Geometry: final body of the model. Coordinates: model frame, mm. A direction names the side the tool comes from. Give positions to 0.01 mm unless a question says otherwise; leave off trailing zeros. Loops run counter-clockwise (first coordinate to the right, second up) from the corner with the lowest first, then second, coordinate; pieces in that order, holes last. Notation, with made-up numbers: (-21, -31.75) -> (-3, -31.75) arc R27 ccw to (-3, -14.75) -> close; hole circle Ø1 at (67, -2.75). An arc over 180 degrees is marked (long way). One line per question, with ' | ' between items. Start each with the question number.
Item 1: Mould query, pull axis Z, two halves, no side actions, for faces 4 (the flat face through (34, -60, -4)), 5 (the flat face through (34, -77, 60)), 6 (the flat face through (50, -9, 1)), 7 (the cylindrical face through (34.255, -77.465, 50.103)). Classes: released by +Z, released by -Z, zero draft, split by the parting line, or undercut.
Item 2: Section C-C on z = 1.5. Return loops of the section in (x, y).
Item 3: Material intervals for line 1 along Z through (x, y) = (56, 8); line 2 along Y through (x, z) = (28.5, 35); line 3 along Z through (x, y) = (57.5, -12.5), sorted ascending. Write a range as [from, to].
Item 4: Set-up query: faces 1 (the flat face through (23.459, -36, 1)), 2 (the flat face through (12, -20, 0)), 3 (the flat face through (21, -39, 3)). Return all of +Z, -Z, +X, -X, +Y, -Y with unobstructed straight access to the full face (end or side cutting, diameter ignored); none if empty.
Item 5: Pin query (flat end, axial travel): P1, Ø15, axis at x = 56.5, y = -14.5, coming from the -Z side; P2, Ø4.5, axis at x = 18.06, y = -3.6, coming from the +Z side; P3, Ø13, axis at x = 33.73, z = 46.14, coming from the +Y side. Return the tip coordinate at first contact, or that it passes through.
Item 6: Section D-D on x = 50. Return loops of the section in (y, z), then the cut area to 3 significant figures.
Item 7: Section A-A on y = -20. Return loops of the section in (x, z), then the cut area to 3 significant figures.
Item 8: Section B-B on y = -3.6. Return loops of the section in (x, z), then the cut area to 3 significant figures.
from build123d import *

# Parameters (mm, degrees)
F0_W     = 10
F0_H     = 10
F0_W_2   = 9
F0_H_2   = 9
F0_R     = 1.75
F0_R_2   = 1.9678984668
F1_DEPTH = 3
F0_W_3   = 59.7
F0_H_3   = 5
F2_DEPTH = 60
F4_D     = 8
F6_DEPTH = 4
F8_D     = 8


# Not quite as in the source:
# - a feature names something its author has since deleted; it is built from what else it names


with BuildPart() as f1:
    # F0 (on Top) → F1 (new body)
    with BuildSketch(Plane.XY):
        with Locations((9.4588409364, 5)):
            Rectangle(F0_W, F0_H)
        with Locations((59.1588409364, 5)):
            Rectangle(F0_W, F0_H)
        Polygon((14.4588409364, 10), (14.4588409364, 0), (23.4588409364, 0), (45.1588409364, 0), (54.1588409364, 0), (54.1588409364, 10), align=None)
        Polygon((14.4588409364, -9), (14.4588409364, 0), (4.4588409364, 0), (4.4588409364, -40), (14.4588409364, -40), (14.4588409364, -31), align=None)
        Polygon((64.1588409364, 0), (54.1588409364, 0), (54.1588409364, -9), (54.1588409364, -31), (54.1588409364, -40), (64.1588409364, -40), align=None)
        Polygon((14.4588409364, -40), (4.4588409364, -40), (4.4588409364, -50), (4.4588409364, -75), (64.1588409364, -75), (64.1588409364, -50), (64.1588409364, -40), (54.1588409364, -40), (45.1588409364, -40), (23.4588409364, -40), align=None)
        with Locations((18.9588409364, -4.5)):
            Rectangle(F0_W_2, F0_H_2)
        with Locations((18.0588409364, -3.6)):
            Circle(F0_R, mode=Mode.SUBTRACT)
        with Locations((49.6588409364, -4.5)):
            Rectangle(F0_W_2, F0_H_2)
        with Locations((50.5588409364, -3.6)):
            Circle(F0_R, mode=Mode.SUBTRACT)
        with Locations((18.9588409364, -35.5)):
            Rectangle(F0_W_2, F0_H_2)
        with Locations((18.2767394032, -36.1821015332)):
            Circle(F0_R_2, mode=Mode.SUBTRACT)
        with Locations((49.6588409364, -35.5)):
            Rectangle(F0_W_2, F0_H_2)
        with Locations((50.5588409364, -36.4)):
            Circle(F0_R, mode=Mode.SUBTRACT)
        Polygon((4.4588409364, 10), (14.4588409364, 10), (54.1588409364, 10), (64.1588409364, 10), (64.1588409364, 15), (4.4588409364, 15), align=None)
    extrude(amount=F1_DEPTH)

    # F0 (on Top) → F2 (join)
    with BuildSketch(Plane.XY):
        with Locations((34.3088409364, -77.5)):
            Rectangle(F0_W_3, F0_H_3)
    extrude(amount=F2_DEPTH)

    # F4 (through all)
    with Locations(Plane.XZ.offset(80)):
        with Locations((33.7338409364, 46.1369195342)):
            Hole(F4_D / 2)

    # F5 (on face) → F6 (join)
    with BuildSketch(Plane(origin=(0, 0, 0), x_dir=(1, 0, 0), z_dir=(0, 0, -1))):
        Polygon((4.4588409364, 40), (23.4588409364, 40), (45.1588409364, 40), (64.1588409364, 40), (64.1588409364, 80), (4.4588409364, 80), align=None)
        Polygon((23.4588409364, 0), (4.4588409364, 0), (4.4588409364, -10), (4.4588409364, -15), (64.1588409364, -15), (64.1588409364, -10), (64.1588409364, 0), (45.1588409364, 0), align=None)
    extrude(amount=F6_DEPTH)

    # F8 (through all)
    with Locations(Plane.XY.offset(3)):
        with Locations((34.1588409364, -55.4992741766)):
            Hole(F8_D / 2)


solid = f1.part
Result sheet:
1) face 4: released by -Z | face 5: released by +Z | face 6: zero draft | face 7: undercut
2) outline: (4.46, -80) -> (64.16, -80) -> (64.16, 15) -> (4.46, 15) -> close; hole (14.46, -31) -> (23.46, -31) -> (23.46, -40) -> (45.16, -40) -> (45.16, -31) -> (54.16, -31) -> (54.16, -9) -> (45.16, -9) -> (45.16, 0) -> (23.46, 0) -> (23.46, -9) -> (14.46, -9) -> close; hole circle Ø3.94 at (18.28, -36.18); hole circle Ø3.5 at (18.06, -3.6); hole circle Ø8 at (34.16, -55.5); hole circle Ø3.5 at (50.56, -36.4); hole circle Ø3.5 at (50.56, -3.6)
3) line 1: z = [-4, 3] | line 2: y = [-80, -75] | line 3: z = [0, 3]
4) face 1: +Z, -Z | face 2: -Z, +X, -X | face 3: +Z, +X, -X, +Y
5) P1: stops at z = 0 | P2: stops at z = 3 | P3: stops at y = -75
6) outline: (-80, -4) -> (-40, -4) -> (-40, 0) -> (-38.06, 0) -> (-38.06, 3) -> (-75, 3) -> (-75, 60) -> (-80, 60) -> close; (-34.74, 0) -> (-31, 0) -> (-31, 3) -> (-34.74, 3) -> close; (-9, 0) -> (-5.26, 0) -> (-5.26, 3) -> (-9, 3) -> close; (-1.94, 0) -> (0, 0) -> (0, -4) -> (15, -4) -> (15, 3) -> (-1.94, 3) -> close | area: 704 mm²
7) outline: (4.46, 0) -> (14.46, 0) -> (14.46, 3) -> (4.46, 3) -> close; (54.16, 0) -> (64.16, 0) -> (64.16, 3) -> (54.16, 3) -> close | area: 60.0 mm²
8) outline: (4.46, 0) -> (16.31, 0) -> (16.31, 3) -> (4.46, 3) -> close; (19.81, 0) -> (23.46, 0) -> (23.46, 3) -> (19.81, 3) -> close; (45.16, 0) -> (48.81, 0) -> (48.81, 3) -> (45.16, 3) -> close; (52.31, 0) -> (64.16, 0) -> (64.16, 3) -> (52.31, 3) -> close | area: 93.0 mm²
